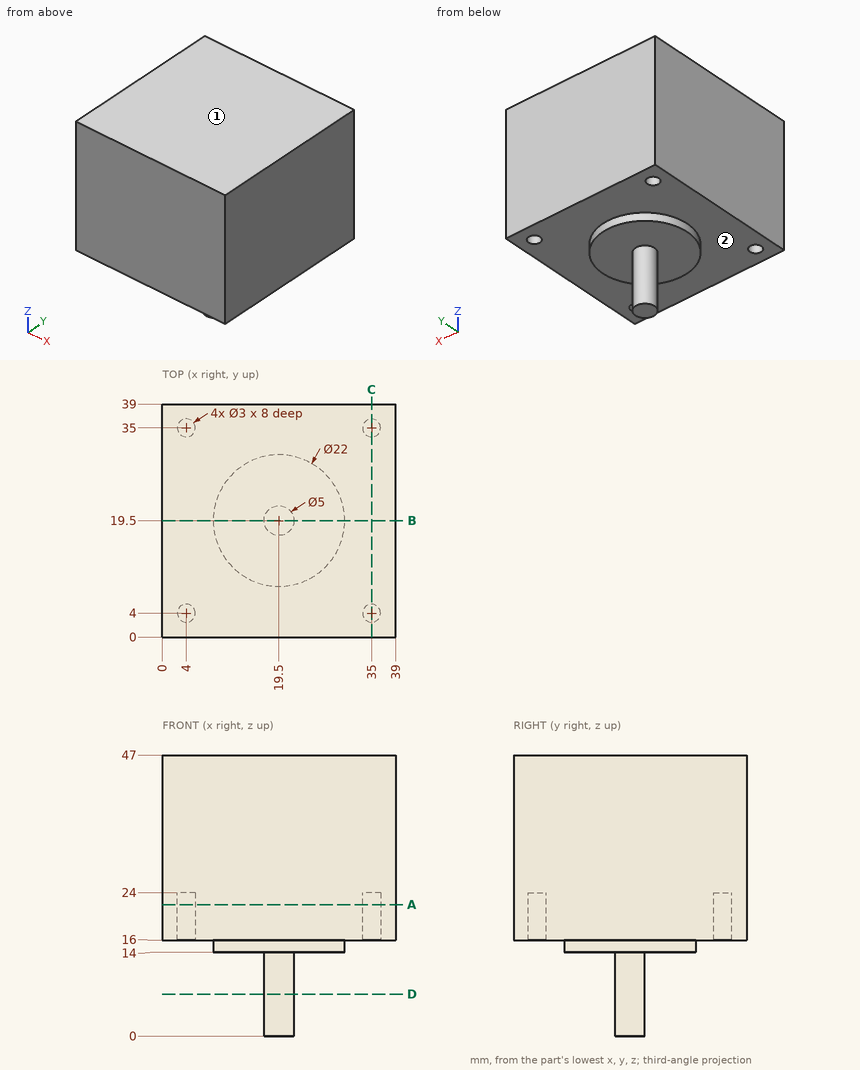
Geometry check sheet. Reference: drawing and pictorial views, mm from the part's lowest x, y, z. A direction names the side the tool comes from. Round coordinates to 2 decimals unless told otherwise and drop trailing zeros. Write each loop counter-clockwise with the first axis right and the second up, starting at its lowest first coordinate (ties: lowest second). Pieces come first, ordered by that corner, then holes.
1. Scan lines: L1, parallel to X at y = 35, z = 20; L2, parallel to X at y = 35.5, z = 20. Record each from-to range of solid material in increasing order.
2. Section check A-A on z = 22. Enter the section's corners in (x, y), plus the area to 3 significant figures.
3. Gauge pin test, flat ends, axial feed: P1, Ø3.5, axis at x = 34.5, y = 4.5, coming from the -Z side; P2, Ø2.5, axis at x = 4, y = 35, coming from the -Z side. Record the tip position at first contact, or that the pin passes through.
4. Section check D-D on z = 7. Enter the section's corners in (x, y), plus the area to 3 significant figures.
5. Section check B-B on y = 19.5. Enter the section's corners in (x, z).
6. Access from +Z, -Z, +X, -X, +Y, -Y to the whole of each face (thin tool, end or side, straight path). Record for the marked faces 1 and 2.
7. Section check C-C on x = 35. Enter the section's corners in (y, z), plus the area to 3 significant figures.
Answer:
1. L1: x = 0 to 2.5, 5.5 to 33.5, 36.5 to 39
1. L2: x = 0 to 2.59, 5.41 to 33.59, 36.41 to 39
2. outline: (0, 0) - (39, 0) - (39, 39) - (0, 39) - close; hole circle Ø3 at (4, 4); hole circle Ø3 at (4, 35); hole circle Ø3 at (35, 4); hole circle Ø3 at (35, 35)
2. area: 1,490 mm2
3. P1: stops at z = 16
3. P2: stops at z = 24
4. outline: circle Ø5 at (19.5, 19.5)
4. area: 19.6 mm2
5. outline: (0, 16) - (8.5, 16) - (8.5, 14) - (17, 14) - (17, 0) - (22, 0) - (22, 14) - (30.5, 14) - (30.5, 16) - (39, 16) - (39, 47) - (0, 47) - close
6. face 1: +Z, +X, -X, +Y, -Y
6. face 2: -Z
7. outline: (0, 16) - (2.5, 16) - (2.5, 24) - (5.5, 24) - (5.5, 16) - (33.5, 16) - (33.5, 24) - (36.5, 24) - (36.5, 16) - (39, 16) - (39, 47) - (0, 47) - close
7. area: 1,160 mm2
